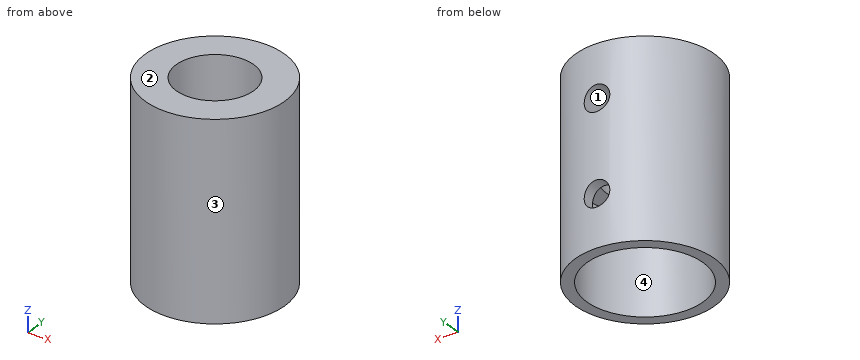
```python
from build123d import *

# Parameters (mm, degrees)
CROQUIS2_R            = 1
CORTAR_EXTRUIR1_DEPTH = 10
CROQUIS3_R            = 3
CORTAR_EXTRUIR2_DEPTH = 7.5
CROQUIS4_R            = 4.5
CORTAR_EXTRUIR3_DEPTH = 7.5


with BuildPart() as part:
    # Croquis1 → Revolución1 (revolve)
    with BuildSketch(Plane(origin=(0, 0, 0), x_dir=(1, 0, 0), z_dir=(0, 1, 0))):
        Polygon((0, -7.5), (0, 0), (0, 7.5), (5.4, 7.5), (5.4, -7.5), align=None)
    revolve(axis=Axis((0, 0, 0), (0, 0, -1)))

    # Croquis2 → Cortar-Extruir1 (cut)
    with BuildSketch(Plane(origin=(0, 0, 0), x_dir=(1, 0, 0), z_dir=(0, 1, 0))):
        with Locations(Location((0, -3.5, 0), (0, 0, 90))):
            Circle(CROQUIS2_R)
        with Locations(Location((0, 3.5, 0), (0, 0, 90))):
            Circle(CROQUIS2_R)
    extrude(amount=CORTAR_EXTRUIR1_DEPTH, mode=Mode.SUBTRACT)

    # Croquis3 → Cortar-Extruir2 (cut)
    with BuildSketch(Plane.XY.offset(7.5)):
        Circle(CROQUIS3_R)
    extrude(amount=-CORTAR_EXTRUIR2_DEPTH, mode=Mode.SUBTRACT)

    # Croquis4 → Cortar-Extruir3 (cut)
    with BuildSketch(Plane(origin=(0, 0, -7.5), x_dir=(-1, 0, 0), z_dir=(0, 0, -1))):
        Circle(CROQUIS4_R)
    extrude(amount=-CORTAR_EXTRUIR3_DEPTH, mode=Mode.SUBTRACT)


solid = part.part
```
Can you work these out from the model? Positions are in its coordinate system, mm. Face numbers are marked on the shaded views. A direction names the side the tool comes from. Give positions to 0.01 mm unless a question says otherwise; leave off trailing zeros. Loops run counter-clockwise (first coordinate to the right, second up) from the corner with the lowest first, then second, coordinate; pieces in that order, holes last. Notation, with made-up numbers: M 60.25,15 L 69.25,15 A9 cw 69.25,31 Z; hole C 42.25,64 d9. An arc over 180 degrees is marked long. Use one line per item in the form item = value. Start each with the question number.
(1) I want a section at D-D, the plane z = 6.25. Write out the boundary of the cut face in (x, y), and give its area (3 significant figures).
(2) I want a section at B-B, the plane x = 0. Write out the boundary of the cut face in (y, z), and give its area (3 significant figures).
(3) I want a section at A-A, the plane y = 0. Write out the boundary of the cut face in (x, z), and give its area (3 significant figures).
(4) Please list where these lines run through material, in increasing order: line 1 (Y direction, x = 0, z = 1); line 2 (Z direction, x = -3.25, y = -0.75); line 3 (Y direction, x = 2.5, z = 2.75).
(5) On a 3-axis mill with a long thin cutter (end or side, diameter ignored), from which of +Z, -Z, +X, -X, +Y, -Y can I reach the whole of each face in a straight line? I mean the marked faces 3 and 4. Say none if no direction works.
(6) Thinking about a two-plate mould opening in Z: for the marked faces 1 and 2, which applies, released by +Z, released by -Z, zero draft, split by the parting line, or undercut?
(7) I want a section at C-C, the plane x = 2.25. Write out the boundary of the cut face in (y, z).
(8) I'm going to push flat-ended pins straight in: P1, Ø1.5, axis at y = 1, z = 1, coming from the +X side; P2, Ø1.6, axis at x = 0, z = -3.5, coming from the +Y side; P3, Ø3, axis at x = -2.5, y = 0.5, coming from the -Z side. Where does each tip first touch, or does it pass through?
Worked out:
q1.outline = C 0,0 d10.8; hole C 0,0 d6
q1.area = 63.3 mm²
q2.outline = M -5.4,-7.5 L -4.5,-7.5 L -4.5,0 L -3,0 L -3,7.5 L -5.4,7.5 Z; M 3,0 L 4.5,0 L 4.5,-2.5 L 5.4,-2.5 L 5.4,2.5 L 3,2.5 Z; M 3,4.5 L 5.4,4.5 L 5.4,7.5 L 3,7.5 Z; M 4.5,-7.5 L 5.4,-7.5 L 5.4,-4.5 L 4.5,-4.5 Z
q2.area = 42.9 mm²
q3.outline = M -5.4,-7.5 L -4.5,-7.5 L -4.5,0 L -3,0 L -3,7.5 L -5.4,7.5 Z; M 3,0 L 4.5,0 L 4.5,-7.5 L 5.4,-7.5 L 5.4,7.5 L 3,7.5 Z
q3.area = 49.5 mm²
q4.line_1 = -5.4 to -3, 3 to 5.4
q4.line_2 = 0 to 7.5
q4.line_3 = -4.79 to -1.66, 1.66 to 4.79
q5.face_3 = +Z, -Z
q5.face_4 = -Z
q6.face_1 = undercut
q6.face_2 = released by +Z
q7.outline = M -4.91,-7.5 L -3.9,-7.5 L -3.9,0 L -1.98,0 L -1.98,7.5 L -4.91,7.5 Z; M 1.98,0 L 3.9,0 L 3.9,-7.5 L 4.91,-7.5 L 4.91,7.5 L 1.98,7.5 Z
q8.P1 = 5.39
q8.P2 = -4.43
q8.P3 = 0
